Verification items for this drawing (mm, ordinates from the low corner). Give positions to 0.01 mm unless a question says otherwise; leave off trailing zeros. Write each loop counter-clockwise with the first axis right and the second up, starting at its lowest first coordinate (ties: lowest second). Pieces come first, ordered by that corner, then holes. Notation, with made-up numbers: (64, 11.5) -> (77, 11.5) arc R10 cw to (77, 17.5) -> close; hole circle Ø9 at (79, 33.25). An arc over 180 degrees is marked (long way). Write item = value, one per line.
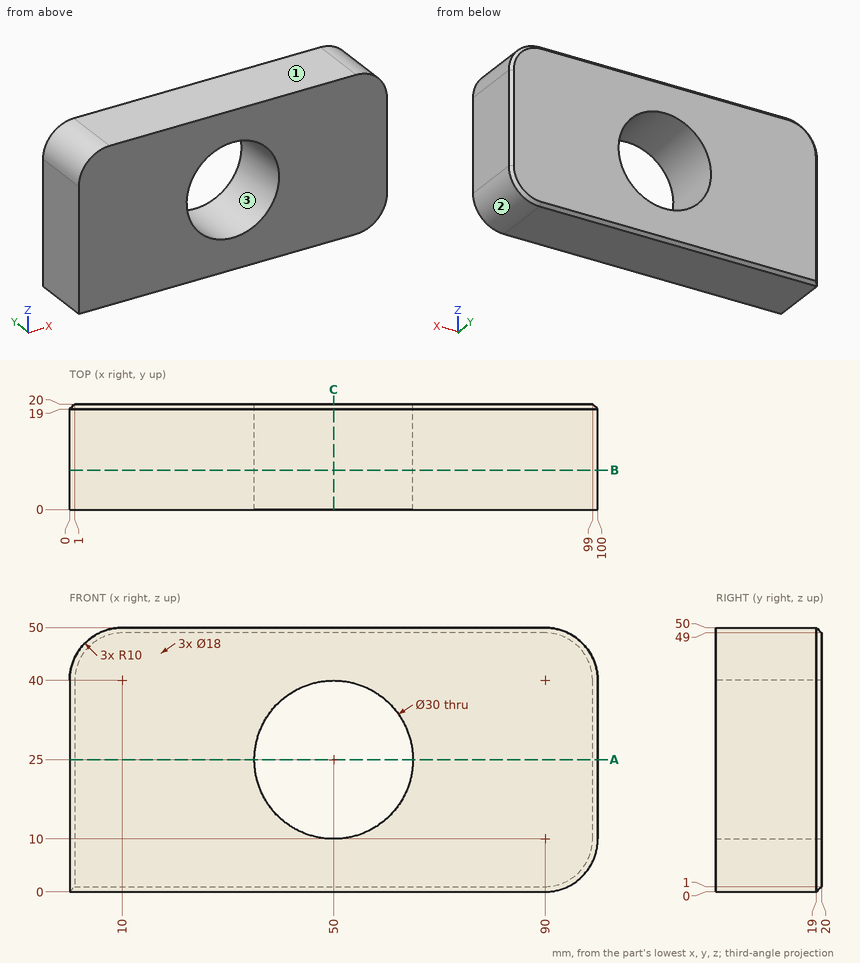
Item 1: Sectioned sample at A-A on z = 25. Record the cut outline in (x, y), then the cut area to 3 significant figures.
Response values:
outline = (0, 0) -> (35, 0) -> (35, 20) -> (1, 20) -> (0, 19) -> close; (65, 0) -> (100, 0) -> (100, 19) -> (99, 20) -> (65, 20) -> close
area = 1,400 mm^2
Item 2: Material ranges on line 1 (X direction, y = 6.75, z = 25); line 2 (X direction, y = 12, z = 29); line 3 (Z direction, x = 45, y = 6.25), recorded low to high.
Response values:
line_1 = 0 to 35, 65 to 100
line_2 = 0 to 35.54, 64.46 to 100
line_3 = 0 to 10.86, 39.14 to 50
Item 3: Sectioned sample at B-B on y = 7.5. Record the cut outline in (x, z).
Response values:
outline = (0, 0) -> (90, 0) arc R10 ccw to (100, 10) -> (100, 40) arc R10 ccw to (90, 50) -> (10, 50) arc R10 ccw to (0, 40) -> close; hole circle Ø30 at (50, 25)
Item 4: Mould release check, pull along Z, two halves, no side actions. Record for the marked faces 1, 2 and 3: +Z half, -Z half, draft (parallel to the pull), parting line (faces both ways), or undercut.
Response values:
face_1 = +Z half
face_2 = -Z half
face_3 = undercut
Item 5: Sectioned sample at C-C on x = 50. Record the cut outline in (y, z), then the cut area to 3 significant figures.
Response values:
outline = (0, 0) -> (19, 0) -> (20, 1) -> (20, 10) -> (0, 10) -> close; (0, 40) -> (20, 40) -> (20, 49) -> (19, 50) -> (0, 50) -> close
area = 399 mm^2
